The model under review builds one solid part; all positions refer to its coordinate system, in mm. Round coordinates to 2 decimals unless told otherwise and drop trailing zeros. Write each loop counter-clockwise with the first axis right and the second up, starting at its lowest first coordinate (ties: lowest second). Pieces come first, ordered by that corner, then holes. Notation, with made-up numbers: (-6.5, 27.25) - (41.5, 27.25) arc R19 cw to (41.5, 57.25) - close; hole circle Ø6 at (73.25, 6.25). An arc over 180 degrees is marked (long way). Return JSON: item names as keys, results as strings.
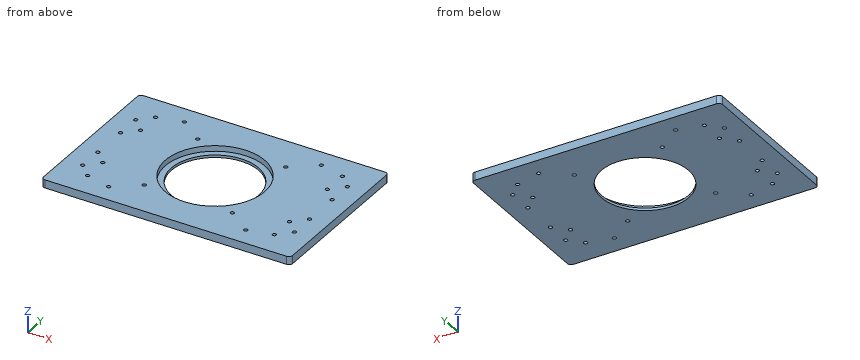
from build123d import *

# Parameters (mm, degrees)
SKETCH_W     = 200
SKETCH_H     = 130
SKETCH_R     = 35
SKETCH_R_2   = 1.5
PAD_DEPTH    = 6.5
SKETCH001_R  = 40
POCKET_DEPTH = 4.5
FILLET_R     = 3


with BuildPart() as part:
    # Sketch → Pad (new body)
    with BuildSketch(Plane.XY):
        with Locations((100, 65)):
            Rectangle(SKETCH_W, SKETCH_H)
        with Locations((100, 65)):
            Circle(SKETCH_R, mode=Mode.SUBTRACT)
        with Locations((45, 115)):
            Circle(SKETCH_R_2, mode=Mode.SUBTRACT)
        with Locations((45, 15)):
            Circle(SKETCH_R_2, mode=Mode.SUBTRACT)
        with Locations((155, 115)):
            Circle(SKETCH_R_2, mode=Mode.SUBTRACT)
        with Locations((155, 15)):
            Circle(SKETCH_R_2, mode=Mode.SUBTRACT)
        with Locations((185, 30)):
            Circle(SKETCH_R_2, mode=Mode.SUBTRACT)
        with Locations((135.353085, 100.338453)):
            Circle(SKETCH_R_2, mode=Mode.SUBTRACT)
        with Locations((64.627773, 29.642413)):
            Circle(SKETCH_R_2, mode=Mode.SUBTRACT)
        with Locations((64.64463, 100.35537)):
            Circle(SKETCH_R_2, mode=Mode.SUBTRACT)
        with Locations((135.352442, 29.63292)):
            Circle(SKETCH_R_2, mode=Mode.SUBTRACT)
        with Locations((175, 20)):
            Circle(SKETCH_R_2, mode=Mode.SUBTRACT)
        with Locations((175, 40)):
            Circle(SKETCH_R_2, mode=Mode.SUBTRACT)
        with Locations((185, 50)):
            Circle(SKETCH_R_2, mode=Mode.SUBTRACT)
        with Locations((175, 90)):
            Circle(SKETCH_R_2, mode=Mode.SUBTRACT)
        with Locations((175, 110)):
            Circle(SKETCH_R_2, mode=Mode.SUBTRACT)
        with Locations((185, 80)):
            Circle(SKETCH_R_2, mode=Mode.SUBTRACT)
        with Locations((185, 100)):
            Circle(SKETCH_R_2, mode=Mode.SUBTRACT)
        with Locations((15, 30)):
            Circle(SKETCH_R_2, mode=Mode.SUBTRACT)
        with Locations((25, 20)):
            Circle(SKETCH_R_2, mode=Mode.SUBTRACT)
        with Locations((25, 40)):
            Circle(SKETCH_R_2, mode=Mode.SUBTRACT)
        with Locations((15, 50)):
            Circle(SKETCH_R_2, mode=Mode.SUBTRACT)
        with Locations((25, 90)):
            Circle(SKETCH_R_2, mode=Mode.SUBTRACT)
        with Locations((25, 110)):
            Circle(SKETCH_R_2, mode=Mode.SUBTRACT)
        with Locations((15, 80)):
            Circle(SKETCH_R_2, mode=Mode.SUBTRACT)
        with Locations((15, 100)):
            Circle(SKETCH_R_2, mode=Mode.SUBTRACT)
    extrude(amount=PAD_DEPTH)

    # Sketch001 (on Face31 of Pad) → Pocket (cut)
    with BuildSketch(Plane.XY.offset(6.5)):
        with Locations((100, 65)):
            Circle(SKETCH001_R)
    extrude(amount=-POCKET_DEPTH, mode=Mode.SUBTRACT)

    # Fillet
    fillet_edges = [part.edges().sort_by_distance(p)[0] for p in [
        (200, 0, 3.25),
        (200, 130, 3.25),
        (0, 0, 3.25),
        (0, 130, 3.25),
    ]]
    fillet(fillet_edges, radius=FILLET_R)


solid = part.part
(1) Add section B-B (x = 72). Write out the cut boundary in (y, z), plus the area to 3 significant figures.
Filled in:
{"outline": "(0, 0) - (44, 0) - (44, 2) - (36.43, 2) - (36.43, 6.5) - (0, 6.5) - close; (86, 0) - (130, 0) - (130, 6.5) - (93.57, 6.5) - (93.57, 2) - (86, 2) - close", "area": "504 mm2"}
(2) Wall thickness on line 1 (Y direction, x = 45, z = 2); line 2 (Y direction, x = 15, z = 4.5); line 3 (Y direction, x = 16, z = 3.75): over which ranges is each line inside the solid? List them lowest first.
Filled in:
{"line 1": "y = 0 to 13.5, 16.5 to 113.5, 116.5 to 130", "line 2": "y = 0 to 28.5, 31.5 to 48.5, 51.5 to 78.5, 81.5 to 98.5, 101.5 to 130", "line 3": "y = 0 to 28.88, 31.12 to 48.88, 51.12 to 78.88, 81.12 to 98.88, 101.12 to 130"}
(3) Add section A-A (y = 65). Write out the cut boundary in (x, z), plus the area to 3 significant figures.
Filled in:
{"outline": "(0, 0) - (65, 0) - (65, 2) - (60, 2) - (60, 6.5) - (0, 6.5) - close; (135, 0) - (200, 0) - (200, 6.5) - (140, 6.5) - (140, 2) - (135, 2) - close", "area": "800 mm2"}
(4) Clearance check with flat-ended pins moving along their axes: pin 1 Ø4 at (x, y) = (185, 50) entering from -Z; pin 2 Ø1.8 at (x, y) = (175, 20) entering from +Z. State where each tip first meets the part, or that it passes through.
Filled in:
{"pin 1": "stops at z = 0", "pin 2": "passes through"}
